Read the model definition and answer for the solid it produces. Units are mm, in the model's axes. Face numbers are marked on the shaded views. A direction names the side the tool comes from. Give positions to 0.01 mm unless a question says otherwise; leave off trailing zeros. Write each loop counter-clockwise with the first axis right and the second up, starting at its lowest first coordinate (ties: lowest second). Pieces come first, ordered by that corner, then holes. Notation, with made-up numbers: M 24,-2.75 L 29,-2.75 A12 ccw 29,12.25 Z; hole C 38.25,39 d8. An arc over 180 degrees is marked long. Put each result on its own line as item: value.
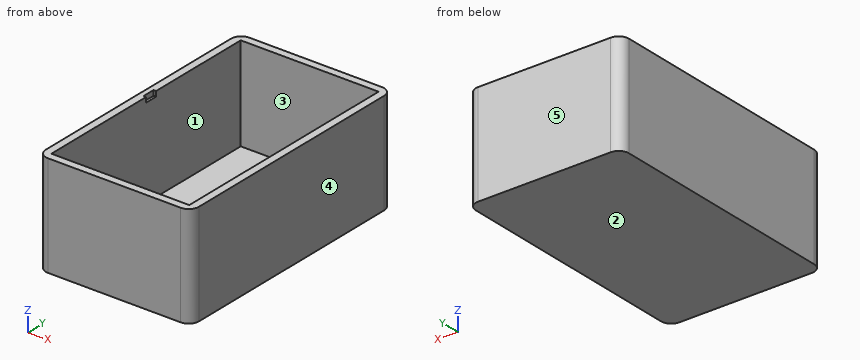
from build123d import *

# Parameters (mm, degrees)
SKETCH_W     = 60
SKETCH_H     = 100
PAD_DEPTH    = 40
THICKNESS_T  = -3
FILLET_R     = 4
SKETCH002_W  = 1
SKETCH002_H  = 2
POCKET_DEPTH = 5


with BuildPart() as part:
    # Sketch → Pad (new body)
    with BuildSketch(Plane.XY):
        Rectangle(SKETCH_W, SKETCH_H)
    extrude(amount=-PAD_DEPTH)

    # Thickness
    thickness_openings = [part.faces().sort_by_distance(p)[0] for p in [
        (0, 0, 0),
    ]]
    offset(amount=THICKNESS_T, openings=thickness_openings, kind=Kind.INTERSECTION)

    # Fillet
    fillet_edges = [part.edges().sort_by_distance(p)[0] for p in [
        (30, -50, -20),
        (-30, -50, -20),
        (30, 50, -20),
        (-30, 50, -20),
    ]]
    fillet(fillet_edges, radius=FILLET_R)

    # Sketch002 → Pocket (cut)
    with BuildSketch(Plane.XZ):
        with Locations((-27.5, -1)):
            Rectangle(SKETCH002_W, SKETCH002_H)
    extrude(amount=-POCKET_DEPTH, mode=Mode.SUBTRACT)


solid = part.part
(1) Section A-A on x = 12.5 is taken. Determine the outline of the cut face in (y, z).
Result:
outline: M -50,-40 L 50,-40 L 50,0 L 47,0 L 47,-37 L -47,-37 L -47,0 L -50,0 Z
(2) Section B-B on z = -8 is taken. Determine the outline of the cut face in (x, y), and give its area (3 significant figures).
Result:
outline: M -30,-46 A4 ccw -26,-50 L 26,-50 A4 ccw 30,-46 L 30,46 A4 ccw 26,50 L -26,50 A4 ccw -30,46 Z; hole M -27,-47 L 27,-47 L 27,47 L -27,47 Z
area: 910 mm²
(3) For a pull along Y with two mould halves and no side action, classify the marked faces 3, 4 and 5 as +Y half, -Y half, draft (parallel to the pull), parting line (faces both ways), or undercut.
Result:
face 3: undercut
face 4: draft
face 5: +Y half
(4) Section C-C on y = -35 is taken. Determine the outline of the cut face in (x, z).
Result:
outline: M -30,-40 L 30,-40 L 30,0 L 27,0 L 27,-37 L -27,-37 L -27,0 L -30,0 Z
(5) Given pin 1 Ø2 at (x, y) = (0.5, 26.5) entering from +Z; pin 2 Ø0.8 at (x, z) = (-27.5, -1) entering from -Y; pin 3 Ø0.8 at (x, y) = (-27.5, 1.5) entering from +Z, each flat-ended and moving along its own axis, determine where each tip first touches the part or whether it passes through.
Result:
pin 1: stops at z = -37
pin 2: stops at y = -49.85
pin 3: stops at z = -2
(6) Straight lines are drawn through the part: line 1 along X through (y, z) = (-40.5, -2); line 2 along Y through (x, z) = (-17, -18.5); line 3 along Z through (x, y) = (21.5, 38.5). For each, find the intervals that lie inside material, in ascending order. Write a range as from..to.
Result:
line 1: x = -30..-27, 27..30
line 2: y = -50..-47, 47..50
line 3: z = -40..-37
(7) Which of the six approach directions +Z, -Z, +X, -X, +Y, -Y give full straight-line access (tool end or side, diameter ignored) to the marked faces 1 and 2?
Result:
face 1: +Z
face 2: -Z, +X, -X, +Y, -Y
